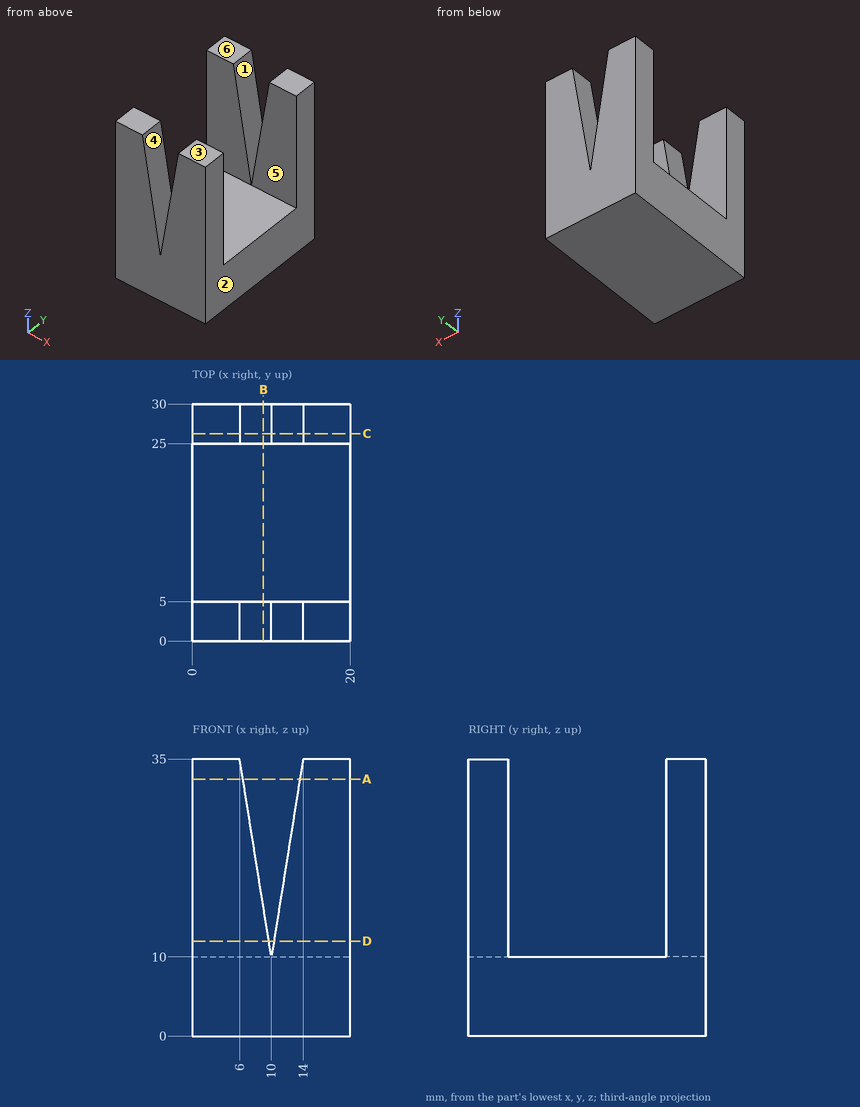
Geometry check sheet. Reference: drawing and pictorial views, mm from the part's lowest x, y, z. A direction names the side the tool comes from. Give positions to 0.01 mm unless a question says otherwise; leave off trailing zeros. Write each loop counter-clockwise with the first axis right and the second up, starting at its lowest first coordinate (ties: lowest second). Pieces come first, ordered by that corner, then holes.
Item 1: Cross-section at D-D (z = 12). Enter the section's corners in (x, y), and give its area (3 significant figures).
Item 2: Scan lines: L1, parallel to Y at x = 19.25, z = 17.5; L2, parallel to Z at x = 11.25, y = 12; L3, parallel to X at y = 4.75, z = 19. Record each from-to range of solid material in increasing order.
Item 3: Cross-section at A-A (z = 32.5). Enter the section's corners in (x, y), and give its area (3 significant figures).
Item 4: Access from +Z, -Z, +X, -X, +Y, -Y to the whole of each face (thin tool, end or side, straight path). Record for the marked faces 4, 5 and 6.
Item 5: Cross-section at C-C (y = 26.25). Enter the section's corners in (x, z), and give its area (3 significant figures).
Item 6: Draft check along X on the marked faces 1, 2 and 3. Enter one of: released by +X, released by -X, zero draft, split by the parting line, or undercut.
Item 7: Gauge pin test, flat ends, axial feed: pin 1 (10 mm diameter, centred on x = 4.5, y = 9, fed in from -Z); pin 2 (5 mm diameter, centred on x = 18, y = 17, fed in from +Z); pin 3 (3 mm diameter, centred on x = 8.5, z = 31, fed in from +Y). Record the tip position at first contact, or that the pin passes through.
Item 8: Cross-section at B-B (x = 9). Enter the section's corners in (y, z), and give its area (4 significant figures).
Report:
1. outline: (0, 0) - (9.68, 0) - (9.68, 5) - (0, 5) - close; (0, 25) - (9.68, 25) - (9.68, 30) - (0, 30) - close; (10.32, 0) - (20, 0) - (20, 5) - (10.32, 5) - close; (10.32, 25) - (20, 25) - (20, 30) - (10.32, 30) - close
1. area: 194 mm2
2. L1: y = 0 to 5, 25 to 30
2. L2: z = 0 to 10
2. L3: x = 0 to 8.56, 11.44 to 20
3. outline: (0, 0) - (6.4, 0) - (6.4, 5) - (0, 5) - close; (0, 25) - (6.4, 25) - (6.4, 30) - (0, 30) - close; (13.6, 0) - (20, 0) - (20, 5) - (13.6, 5) - close; (13.6, 25) - (20, 25) - (20, 30) - (13.6, 30) - close
3. area: 128 mm2
4. face 4: +Z, +Y, -Y
4. face 5: +Z, +X, -X
4. face 6: +Z, +X, -X, +Y, -Y
5. outline: (0, 0) - (20, 0) - (20, 35) - (14, 35) - (10, 10) - (6, 35) - (0, 35) - close
5. area: 600 mm2
6. face 1: undercut
6. face 2: released by +X
6. face 3: zero draft
7. pin 1: stops at z = 0
7. pin 2: stops at z = 10
7. pin 3: passes through
8. outline: (0, 0) - (30, 0) - (30, 16.25) - (25, 16.25) - (25, 10) - (5, 10) - (5, 16.25) - (0, 16.25) - close
8. area: 362.5 mm2
